For this review, use the dimensioned drawing (mm, ordinates from the lowest corner) and the shaded views. A direction names the side the tool comes from. Coordinates: 2 decimals unless noted, no trailing zeros. Order: outer loops, then holes, each group sorted by start corner. A loop starts at its lowest first (then second) coordinate and runs counter-clockwise, first axis right, second up. Notation, with made-up numbers: M 52,7 L 81,7 A14 ccw 81,28 Z; hole C 9,-30 d7. An arc over 180 degrees is marked long. One line per item, written item: value.
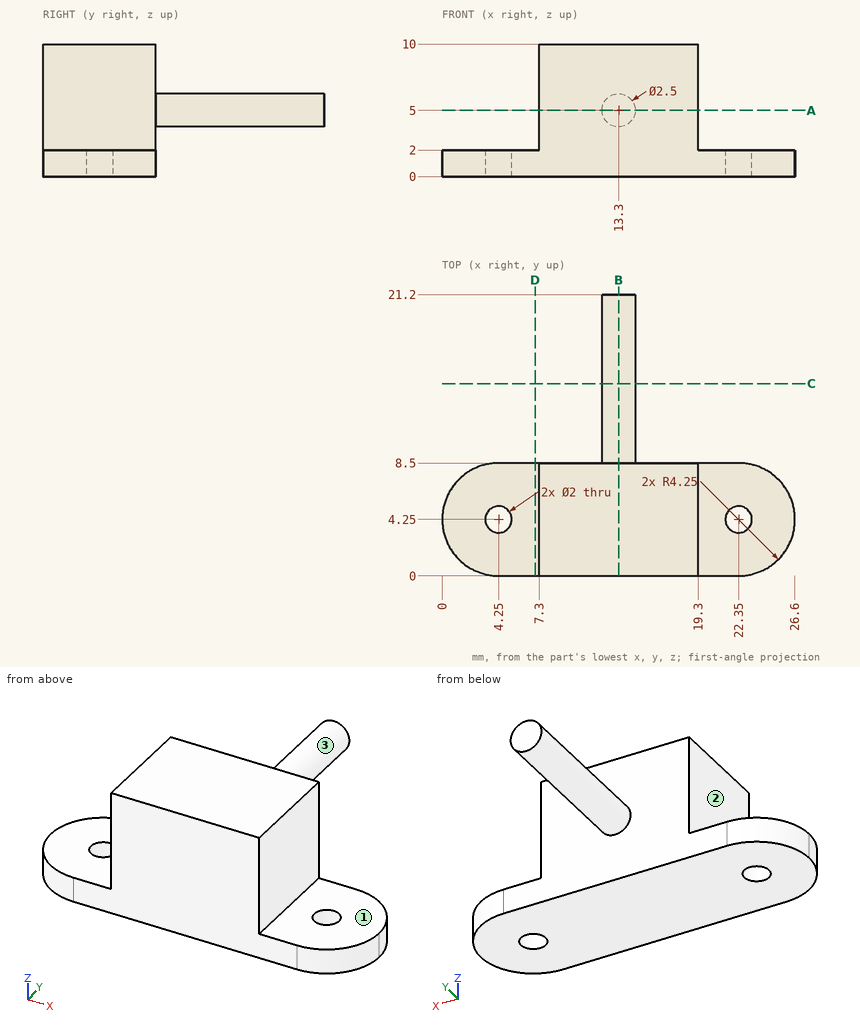
(1) We need section D-D, the plane x = 7. State the section outline as (y, z) points, plus the area to 3 significant figures.
Geometry results:
outline: M 0,0 L 8.5,0 L 8.5,2 L 0,2 Z
area: 17.0 mm2
(2) For L1, parallel to Y at x = 18, z = 9.75; L2, parallel to Z at x = 19.5, y = 6.75; L3, parallel to X at y = 7.25, z = 2.25, list the stretches that pass through material, from the lowest coordinate up.
Geometry results:
L1: y = 0 to 8.5
L2: z = 0 to 2
L3: x = 7.3 to 19.3
(3) Tool access review of the marked faces 1, 2 and 3: name each direction out of +Z, -Z, +X, -X, +Y, -Y from which nothing blocks a thin tool from reaching the whole face with its end or side.
Geometry results:
face 1: +Z, +X, +Y, -Y
face 2: +Z, -X, +Y, -Y
face 3: +Y
(4) We need section B-B, the plane x = 13.3. State the section outline as (y, z) points, plus the area to 3 significant figures.
Geometry results:
outline: M 0,0 L 8.5,0 L 8.5,3.75 L 21.2,3.75 L 21.2,6.25 L 8.5,6.25 L 8.5,10 L 0,10 Z
area: 117 mm2
(5) We need section A-A, the plane z = 5. State the section outline as (x, y) points.
Geometry results:
outline: M 7.3,0 L 19.3,0 L 19.3,8.5 L 14.55,8.5 L 14.55,21.2 L 12.05,21.2 L 12.05,8.5 L 7.3,8.5 Z
(6) Insertion check: pin 1 Ø4 at (y, z) = (5.5, 4.5) entering from -X; pin 2 Ø8 at (x, y) = (24, 2) entering from +Z; pin 3 Ø6 at (y, z) = (8.5, 3) entering from -X. Each pin has a flat end and moves straight along its axis. Give the tip position at first contact, or say it passes through.
Geometry results:
pin 1: stops at x = 7.3
pin 2: stops at z = 2
pin 3: stops at x = 0.24
(7) We need section C-C, the plane y = 14.5. State the section outline as (x, z) points, plus the area to 3 significant figures.
Geometry results:
outline: C 13.3,5 d2.5
area: 4.91 mm2
